Autodesk Inventor part; units mm, degrees
ref_plane "YZ Plane" through (0, 0, 0) normal (1, 0, 0) x (0, 1, 0)
ref_plane "XZ Plane" through (0, 0, 0) normal (0, 1, 0) x (-1, 0, 0)
ref_plane "XY Plane" through (0, 0, 0) normal (0, 0, 1) x (1, 0, 0)
sketch "Skizze1" plane through (0, 0, 0) normal (0, 0, 1) x (1, 0, 0)
  line L0 (0, 0) -> (0, 4)
  line L1 (0, 4) -> (12.5, 4)
  line L2 (12.5, 4) -> (12.5, 6)
  line L3 (12.5, 6) -> (48.5, 6)
  line L4 (48.5, 6) -> (48.5, 4)
  line L5 (48.5, 4) -> (61, 4)
  line L6 (61, 4) -> (61, 0)
  line L7 (61, 0) -> (0, 0)
  dimension "d1" = 12.5
  dimension "d2" = 12.5
  dimension "d3" = 8
  dimension "d4" = 12
  dimension "d29" = 36
revolve "Umdrehung1" add sketch "Skizze1" angle 360 about axis through (61, 0, 0) along (-1, 0, 0)
sketch "Skizze2" plane through (0, 0, 0) normal (-1, 0, 0) x (0, 0, 1)
  point P0 (0, 0)
  point P1 (0, 0)
sketch "Skizze3" plane through (61, 0, 0) normal (1, 0, 0) x (0, 0, -1)
  point P0 (0, 0)
  point P1 (0, 0)
hole "Bohrung1" at (61, 0, 0) direction (-1, 0, 0) diameter 3.242 depth 9 tip angle 118
hole "Bohrung2" at (0, 0, 0) direction (1, 0, 0) diameter 3.242 depth 9 tip angle 118
chamfer "Fase1" distance 0.5 angle 45 4 edges at (0, -4, 0) (61, -4, 0) (61, 0, 1.621) (0, 0, -1.621)
chamfer "Fase2" distance 0.1 angle 45 2 edges at (48.5, -6, 0) (12.5, -6, 0)
ref_plane "Arbeitsebene1" through (30.5, 0, 0) normal (-1, 0, 0) x (0, 0, 1)
equation "\"d1\" = d2"
equation "\"d29\" = MainAxis_Schluesselweite + 2 * ParallelMecha_Bearing_Step_Thickness"
equation "\"ParallelLink_BearingStep_Height\" = 5"
equation "\"ParallelMech_Distance_Step2Flat\" = 14"
equation "\"ParallelLink_Lever_Thickness_1\" = 8"
equation "\"ParallelMecha_Bearing_Step_Thickness\" = 6"
properties part number "ParallelSystem_ProximalPart_Querstreben_v2_Rillenkugellager" material "Edelstahl"
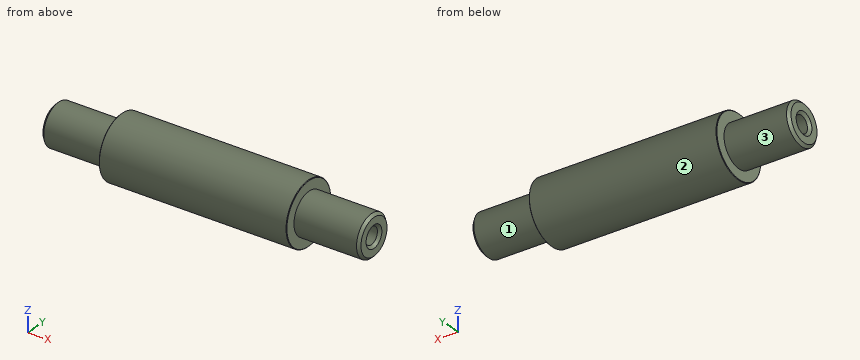
Here's how the part is built. I have some questions about the finished solid (model axes, mm). Face numbers are marked on the shaded views. A direction names the side the tool comes from. Round coordinates to 2 decimals unless told otherwise and drop trailing zeros. Order: outer loops, then holes, each group sorted by start corner. A loop starts at its lowest first (then second) coordinate and runs counter-clockwise, first axis right, second up. Notation, with made-up numbers: (14, 29) -> (71, 29) arc R28 cw to (71, 61) -> close; hole circle Ø6 at (-34.75, 69.25). An arc over 180 degrees is marked (long way). Use a Markdown table: item, result. Add a question column.
(1) I need wall thicknesses on line 1 along Z through (x, y) = (6, 0); line 2 along X through (y, z) = (-1.25, -5.5). Which ranges of each line are inside material? Lowest first, please.
(2) Suppose I cut it at A-A, the plane x = 53.5. Please give me the cut outline in (y, z).
(3) For pin 1 Ø1.5 at (x, z) = (54.5, -0.5) entering from +Y; pin 2 Ø1 at (x, z) = (9.5, -2.5) entering from -Y; pin 3 Ø2 at (x, y) = (23.5, 2) entering from +Z, each with a flat end and sliding along its axis, tell me the tip position at first contact or that it passes through.
(4) For the marked faces 1, 2 and 3, which set-ups out of +Z, -Z, +X, -X, +Y, -Y let a thin tool reach every point of the face, with its end or its side?
(5) Suppose I cut it at B-B, the plane x = 43. Please give me the cut outline in (y, z), and give its area (3 significant figures).
Verdict:
| question | item | result |
|---|---|---|
| 1 | line 1 | -4 to -1.62, 1.62 to 4 |
| 1 | line 2 | 12.5 to 48.5 |
| 2 | outline | circle Ø8 at (0, 0); hole circle Ø3.24 at (0, 0) |
| 3 | pin 1 | y = 4 |
| 3 | pin 2 | y = -3.46 |
| 3 | pin 3 | z = 5.92 |
| 4 | face 1 | +X |
| 4 | face 2 | +X, -X |
| 4 | face 3 | -X |
| 5 | outline | circle Ø12 at (0, 0) |
| 5 | area | 113 mm2 |
